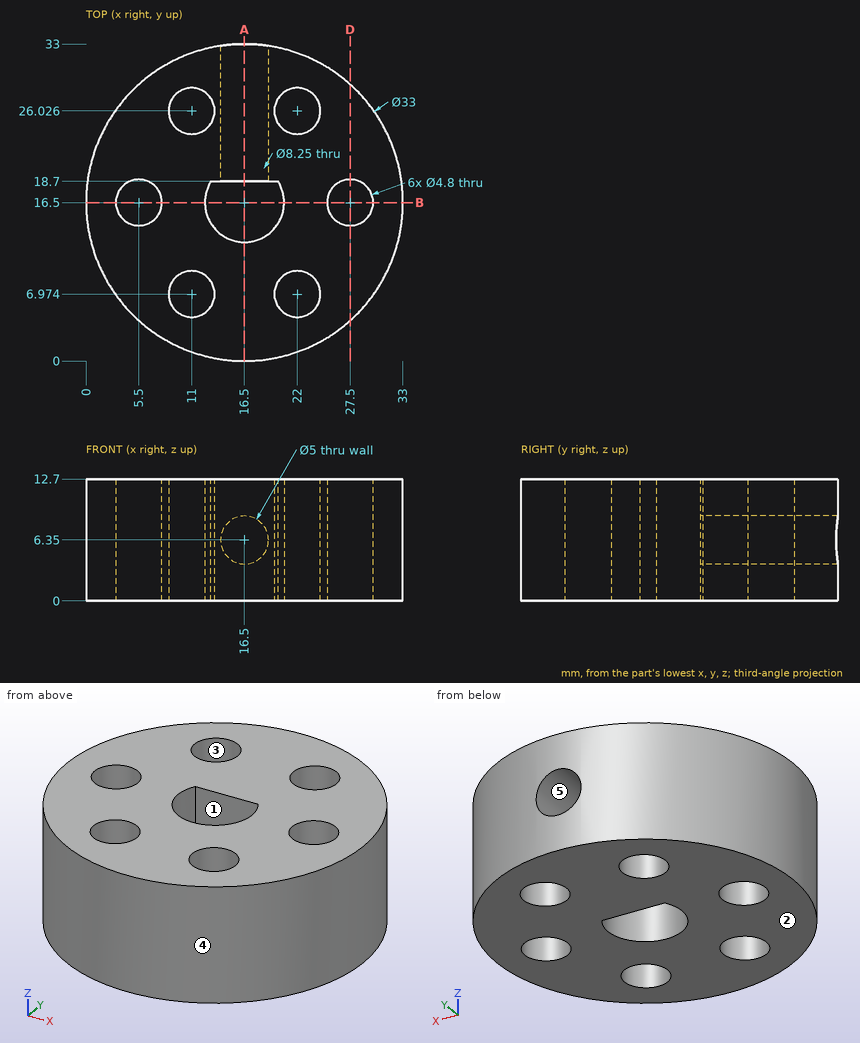
Study the drawing (mm; zero at the part's minimum x, y, z) and answer. A direction names the side the tool comes from. Round coordinates to 2 decimals unless told otherwise and drop trailing zeros. Loops run counter-clockwise (first coordinate to the right, second up) from the corner with the lowest first, then second, coordinate; pieces in that order, holes last. Notation, with made-up numbers: (73, 43) -> (122, 43) arc R24 cw to (122, 64) -> close; hole circle Ø1 at (-36, 74.5). An arc over 180 degrees is marked (long way). One line per item, written item: value.
1) A cutting plane is placed at A-A (x = 16.5). Give the number of separate pieces and of enclosed holes in the cut face, and give its area (3 significant figures).
Answer list:
separate pieces: 3
enclosed holes: 0
area: 267 mm²
2) For the marked faces 1 and 2, determine the directions among +Z, -Z, +X, -X, +Y, -Y from which every point of the face is accessible in a straight line to the end or side of a thin tool.
Answer list:
face 1: +Z, -Z
face 2: -Z, +X, -X, +Y, -Y
3) A cutting plane is placed at D-D (x = 27.5). Determine the outline of the cut face in (y, z), and give its area (3 significant figures).
Answer list:
outline: (4.2, 0) -> (14.1, 0) -> (14.1, 12.7) -> (4.2, 12.7) -> close; (18.9, 0) -> (28.8, 0) -> (28.8, 12.7) -> (18.9, 12.7) -> close
area: 251 mm²
4) A cutting plane is placed at B-B (y = 16.5). Determine the outline of the cut face in (x, z) (1 decimal), and give its area (3 significant figures).
Answer list:
outline: (0, 0) -> (3.1, 0) -> (3.1, 12.7) -> (0, 12.7) -> close; (7.9, 0) -> (12.4, 0) -> (12.4, 12.7) -> (7.9, 12.7) -> close; (20.6, 0) -> (25.1, 0) -> (25.1, 12.7) -> (20.6, 12.7) -> close; (29.9, 0) -> (33, 0) -> (33, 12.7) -> (29.9, 12.7) -> close
area: 192 mm²
5) Flat-ended cylindrical pins translate along their axes: P1, Ø4, axis at x = 22, y = 26.03, coming from the +Z side; P2, Ø6, axis at y = 26, z = 7, coming from the +X side; P3, Ø1, axis at y = 13, z = 3.5, coming from the +X side (1 decimal); P4, Ø1, axis at y = 22.5, z = 9.5, coming from the +X side. Find the tip coordinate at first contact, or state that the pin passes through.
Answer list:
P1: passes through
P2: stops at x = 31.67
P3: stops at x = 32.7
P4: stops at x = 32.06
6) Consider L1, parallel to X at y = 27, z = 2.5 (1 decimal); L2, parallel to Y at x = 21, z = 11 (1 decimal); L3, parallel to X at y = 27, z = 7 (1 decimal). Determine where each line is inside the solid, lowest interval first. Write a range as [from, to].
Answer list:
L1: x = [3.8, 8.8], [13.2, 19.8], [24.2, 29.2]
L2: y = [0.6, 4.8], [9.2, 23.8], [28.2, 32.4]
L3: x = [3.8, 8.8], [13.2, 14.1], [18.9, 19.8], [24.2, 29.2]
7) The mould has two halves that part along Y. Classify the marked faces 3, 4 and 5: pulls with the +Y half, pulls with the -Y half, needs draft (parallel to the pull), parting line crosses it, or undercut.
Answer list:
face 3: undercut
face 4: parting line crosses it
face 5: needs draft
